Input: part model. Units: mm. Frame: model coordinates. A direction names the side the tool comes from. Give positions to 0.01 mm unless a question says otherwise; leave off trailing zeros. Write each loop counter-clockwise with the first axis right and the second up, starting at its lowest first coordinate (ties: lowest second). Pieces come first, ordered by that corner, then holes. Notation, with made-up numbers: (-4.5, 35) - (9.5, 35) arc R35 cw to (9.5, 67) - close; hole circle Ø2 at (33.25, 76.25). An arc over 180 degrees is marked (long way). Answer as CSV lines item,"result". Start each with the question number.
from build123d import *

# Parameters (mm, degrees)
BOSS_EXTRUDE1_DEPTH = 100
CUT_EXTRUDE1_DEPTH  = 50
SKETCH3_R           = 65
BOSS_EXTRUDE2_DEPTH = 20
SKETCH4_R           = 50
BOSS_EXTRUDE3_DEPTH = 40
CHAMFER1_SIZE       = 5
SKETCH5_R           = 5
CUT_EXTRUDE2_DEPTH  = 337.489227168
FILLET1_R           = 5
SKETCH6_R           = 50
CUT_EXTRUDE3_DEPTH  = 337.489227168


with BuildPart() as part:
    # Sketch1 → Boss-Extrude1 (new, symmetric)
    with BuildSketch(Plane.XY):
        with BuildLine():
            Line((0, 75), (-200, 75))
            Line((-200, 75), (-200, -75))
            Line((-200, -75), (0, -75))
            ThreePointArc((0, -75), (75, 0), (0, 75))
        make_face()
    extrude(amount=BOSS_EXTRUDE1_DEPTH, both=True)

    # Sketch2 → Cut-Extrude1 (cut, symmetric)
    with BuildSketch(Plane.XY):
        with BuildLine():
            Line((0, 75), (-100, 75))
            Line((-100, 75), (-100, -75))
            Line((-100, -75), (0, -75))
            ThreePointArc((0, -75), (75, 0), (0, 75))
        make_face()
    extrude(amount=CUT_EXTRUDE1_DEPTH, both=True, mode=Mode.SUBTRACT)

    # Sketch3 → Boss-Extrude2 (add)
    with BuildSketch(Plane.ZY.offset(200)):
        with Locations(Location((0, 0, 0), (0, 0, 180))):
            Circle(SKETCH3_R)
    extrude(amount=BOSS_EXTRUDE2_DEPTH)

    # Sketch4 → Boss-Extrude3 (add)
    with BuildSketch(Plane.ZY.offset(220)):
        Circle(SKETCH4_R)
    extrude(amount=BOSS_EXTRUDE3_DEPTH)

    # Chamfer1
    chamfer1_edges = [part.edges().sort_by_distance(p)[0] for p in [
        (-220, 0, 65),
    ]]
    chamfer(chamfer1_edges, length=CHAMFER1_SIZE)

    # Sketch5 → Cut-Extrude2 (cut, through all)
    with BuildSketch(Plane.XY.offset(100)):
        with Locations((0, 62.5)):
            Circle(SKETCH5_R)
        with Locations((62.5, 0)):
            Circle(SKETCH5_R)
        with Locations((0, -62.5)):
            Circle(SKETCH5_R)
    extrude(amount=-CUT_EXTRUDE2_DEPTH, mode=Mode.SUBTRACT)

    # Fillet1
    fillet1_edges = [part.edges().sort_by_distance(p)[0] for p in [
        (-200, 0, 100),
        (-100, -75, 100),
        (-100, -75, 0),
        (-100, 75, 0),
        (-200, 0, 65),
        (-220, 0, -50),
        (75, 0, 100),
        (-100, -75, -100),
        (-200, 0, -100),
        (-100, 75, -100),
        (75, 0, -100),
        (-100, 75, 100),
        (-200, -75, 0),
        (-200, 75, 0),
    ]]
    fillet(fillet1_edges, radius=FILLET1_R - 0.0001)  # a hair under: the kernel refuses the full size

    # Sketch6 → Cut-Extrude3 (cut, through all)
    with BuildSketch(Plane.XY.offset(100)):
        Circle(SKETCH6_R)
    extrude(amount=-CUT_EXTRUDE3_DEPTH, mode=Mode.SUBTRACT)


solid = part.part
1) Contact query for flat-ended pins moving along their axis: P1, Ø6, axis at x = 0, y = -62.5, coming from the -Z side; P2, Ø2, axis at y = 55, z = 79, coming from the +X side; P3, Ø4, axis at y = 24.5, z = -24, coming from the +X side; P4, Ø2, axis at y = -38.5, z = -62, coming from the -X side. Output: stop coordinate, or through.
2) Cut plane B-B on x = -62.5. Output: boundary loops of the cut face in (y, z), and give its area (3 significant figures).
3) Reachability of faces 5 (the flat face through (-220, 49, -26)), 6 (the flat face through (-100, 1, 1)), 7 (the cylindrical face through (74.98, -1.65, -72.19)) from +Z, -Z, +X, -X, +Y, -Y: full face, straight path, thin tool, end or side. Return the list, or none.
4) Cut plane D-D on x = -19.5. Output: boundary loops of the cut face in (y, z), and give its area (3 significant figures).
5) Pull-direction query (X, two-part tool) for faces 1 (the conical face through (-219.757, 53.446, -27.798)), 2 (the cylindrical face through (47.69, 15.02, 75.35)), 3 (the flat face through (-118, 75, 1)), 4 (the cylindrical face through (57.505, 0.22, 75.35)); classes: +X half, -X half, draft (parallel to the pull), parting line (faces both ways), or undercut.
6) Cut plane A-A on z = 79.5. Output: boundary loops of the cut face in (x, y), and give its area (3 significant figures).
7) Material intervals for line 1 (Y direction, x = 0, z = -76); line 2 (X direction, y = 0.5, z = 73); line 3 (Z direction, x = -32.5, y = -68), sorted ascending. Write a range as from..to.
Numbers:
1,P1,"passes through"
1,P2,"stops at x = 52.05"
1,P3,"stops at x = -100"
1,P4,"stops at x = -200"
2,outline,"(-75, -95) arc R5 ccw to (-70, -100) - (70, -100) arc R5 ccw to (75, -95) - (75, -50) - (-75, -50) - close; (-75, 50) - (75, 50) - (75, 95) arc R5 ccw to (70, 100) - (-70, 100) arc R5 ccw to (-75, 95) - close"
2,area,"15,000 mm²"
3,face 5,"-X"
3,face 6,"+X, +Y, -Y"
3,face 7,"+Z, -Z, +X"
4,outline,"(-75, -95) arc R5 ccw to (-70, -100) - (-46.04, -100) - (-46.04, -50) - (-75, -50) - close; (-75, 50) - (-46.04, 50) - (-46.04, 100) - (-70, 100) arc R5 ccw to (-75, 95) - close; (46.04, -100) - (70, -100) arc R5 ccw to (75, -95) - (75, -50) - (46.04, -50) - close; (46.04, 50) - (75, 50) - (75, 95) arc R5 ccw to (70, 100) - (46.04, 100) - close"
4,area,"5,770 mm²"
5,face 1,"-X half"
5,face 2,"undercut"
5,face 3,"draft"
5,face 4,"undercut"
6,outline,"(-200, -70) arc R5 ccw to (-195, -75) - (0, -75) arc R75 ccw to (0, 75) - (-195, 75) arc R5 ccw to (-200, 70) - close; hole circle Ø100 at (0, 0); hole circle Ø10 at (0, -62.5); hole circle Ø10 at (0, 62.5); hole circle Ø10 at (62.5, 0)"
6,area,"30,700 mm²"
7,line 1,"y = -75..-67.5, -57.5..-50, 50..57.5, 67.5..75"
7,line 2,"x = -200..-50, 50..57.53, 67.47..75"
7,line 3,"z = -100..-50, 50..100"
